Geometry: final body of the model. Coordinates: model frame, mm. A direction names the side the tool comes from. Round coordinates to 2 decimals unless told otherwise and drop trailing zeros. Write each loop counter-clockwise with the first axis right and the second up, starting at its lowest first coordinate (ties: lowest second). Pieces come first, ordered by that corner, then holes. Notation, with made-up numbers: M 6,59.5 L 41,59.5 A33 cw 41,88.5 Z; hole C 79.5,26 d5. An arc over 180 degrees is marked long. Answer as CSV lines item,"result". Start each with the question number.
Q1. Section query D-D on x = 121.5. Output: boundary loops of the cut face in (y, z), and give its area (3 significant figures).
Q2. Section query A-A on z = -21. Output: boundary loops of the cut face in (x, y) (3 decimals), and give its area (3 significant figures).
Q3. Ray query, probe 1 along Z at (x, y) = (28.5, 13); probe 2 along Z at (x, y) = (79, 8.5); probe 3 along Z at (x, y) = (153.5, 21.5). Return the intervals inside material, ascending.
Q4. Reachability of faces 1 (the cylindrical face through (196.46, 3.22, -65.56)), 2 (the flat face through (27, 13, -69.85)) from +Z, -Z, +X, -X, +Y, -Y: full face, straight path, thin tool, end or side. Return the list, or none.
Q5. Mould query, pull axis Z, two halves, no side actions, for faces 3 (the flat face through (92, 13, -76.2)), 4 (the cylindrical face through (-4.404, 18.783, 4.502)), 5 (the flat face through (121, 0, -66)), 6 (the cylindrical face through (183.17, 3.22, -64.18)). Classes: pulls with the +Z half, pulls with the -Z half, needs draft (parallel to the pull), parting line crosses it, or undercut.
Q6. First-contact query: pin 1 (1.5 mm diameter, centred on x = 143.5, z = -72.5, fed in from +Y); pin 2 (1.5 mm diameter, centred on x = 122, z = -76.5, fed in from +Y). Flat tips, straight axial feed; report the tip coordinate or a pass-through.
Q7. Section query C-C on x = 206. Output: boundary loops of the cut face in (y, z), and give its area (3 significant figures).
Autodesk Inventor part; units mm, degrees
ref_plane "YZ Plane" through (0, 0, 0) normal (1, 0, 0) x (0, 1, 0)
ref_plane "XZ Plane" through (0, 0, 0) normal (0, 1, 0) x (-1, 0, 0)
ref_plane "XY Plane" through (0, 0, 0) normal (0, 0, 1) x (1, 0, 0)
sketch "Sketch1" plane through (0, 0, 0) normal (0, 1, 0) x (-1, 0, 0)
  line L0 (0, 0) -> (-238.125, 0)
  line L1 (-238.125, 0) -> (-238.125, -133.35)
  line L2 (-238.125, -133.35) -> (0, -133.35)
  line L3 (0, -133.35) -> (0, 0)
  line L4 (0, 6.35) -> (-237.998, 6.35)
  line L5 (-244.475, -0.127) -> (-244.475, -133.35)
  line L6 (-238.125, -139.7) -> (-0.1245, -139.7)
  line L7 (6.35, -133.35) -> (6.35, 0)
  arc A0 (-0.1245, -139.7) -> (6.35, -133.35) centre (-0.1245, -133.2243) ccw
  arc A1 (6.35, 0) -> (-0.1245, 6.35) centre (-0.1258, -0.127) ccw
  arc A2 (-244.475, -133.2243) -> (-238.125, -139.7) centre (-237.998, -133.2242) ccw
  arc A3 (-237.998, 6.35) -> (-244.475, -0.127) centre (-237.998, -0.127) ccw
  dimension "d0" = 238.125
  dimension "d1" = 133.35
  dimension "d2" = 6.35
  dimension "d9" = 6.477
  dimension "d10" = 6.477
  dimension "d11" = 6.477
extrude "Extrusion1" add sketch "Sketch1" along normal blind 38.1
sketch "Sketch2" plane through (0, 0, 0) normal (0, -1, 0) x (1, 0, 0)
  line L0 (0, 0) -> (238.125, 0)
  line L1 (238.125, 0) -> (238.125, -133.35)
  line L2 (238.125, -133.35) -> (0, -133.35)
  line L3 (0, -133.35) -> (0, 0)
  dimension "d5" = 238.125
  dimension "d6" = 133.35
extrude "Extrusion2" add sketch "Sketch2" against normal blind 6.35
sketch "Sketch7" plane through (0, 6.35, 0) normal (0, 1, 0) x (1, 0, 0)
  line L0 (237.998, 0) -> (155.448, 0)
  line L1 (238.125, 0) -> (0, 0)
  line L2 (155.448, 0) -> (155.448, 57.15)
  line L3 (155.448, 57.15) -> (237.998, 57.15)
  circle A0 centre (218.3382, 65.3946) radius 3.175
  circle A1 centre (199.6313, 65.4249) radius 3.175
  line L4 (218.3382, 65.3946) -> (180.2382, 65.3946)
  circle A2 centre (180.2382, 65.3946) radius 3.175
  dimension "d31" = 82.55
  dimension "d32" = 57.15
  dimension "d33" = 6.35
  dimension "d36" = 6.35
  dimension "d37" = 38.1
  dimension "d38" = 6.35
extrude "Extrusion4" cut sketch "Sketch7" against normal blind 6.35
sketch "Sketch11" plane through (0, 6.35, 0) normal (0, 1, 0) x (1, 0, 0)
  line L0 (57.15, 78.6953) -> (0, 78.6953)
  line L1 (47.625, 76.2) -> (127, 76.2)
  line L2 (47.625, 76.2) -> (127, 76.2)
  line L3 (127, 76.2) -> (127, 63.5)
  line L4 (127, 63.5) -> (47.625, 63.5)
  line L5 (47.625, 63.5) -> (47.625, 76.2)
  line L6 (114.4338, 63.5) -> (127.1338, 63.5)
  line L7 (127.1338, 63.5) -> (127.1338, 0)
  line L8 (127.1338, 0) -> (114.4338, 0)
  line L9 (114.4338, 0) -> (114.4338, 63.5)
  line L10 (238.125, 0) -> (0, 0)
  line L11 (0, 0) -> (0, 82.55)
  line L12 (0, 0) -> (0, 133.35)
  line L13 (0, 82.55) -> (57.15, 82.55)
  line L14 (57.15, 82.55) -> (57.15, 0)
  line L15 (0, 78.6953) -> (47.625, 78.6953)
  line L16 (47.625, 78.6953) -> (47.625, 69.85)
  line L17 (47.625, 69.85) -> (0, 69.85)
  line L18 (0, 69.85) -> (0, 78.6953)
  line L19 (57.15, 78.6953) -> (0, 78.6953)
  line L20 (0, 78.6953) -> (0, 85.0453)
  line L21 (0, 85.0453) -> (57.15, 85.0453)
  line L22 (57.15, 85.0453) -> (57.15, 78.6953)
  point P0 (0, 97.7453)
  point P1 (0, 69.85)
  dimension "d59" = 79.375
  dimension "d60" = 12.7
  dimension "d61" = 12.7
  dimension "d62" = 63.5
  dimension "d70" = 82.55
  dimension "d71" = 6.35
extrude "Extrusion7" add sketch "Sketch11" along normal blind 12.7 contours L0 L11 L13 L14 | L16 L5 L17 L11 L0 | L13 L12 L21 L22 | L14 L4 L5 L1 | L1 L3 L4 L14 | L6 L7 L8 L9 L4
sketch "Sketch12" plane through (0, 6.35, 0) normal (0, 1, 0) x (1, 0, 0)
  line L0 (238.125, 0) -> (0, 0)
  line L1 (238.125, 0) -> (155.575, 0)
  line L2 (151.6176, 0) -> (151.6176, 57.15)
  line L3 (155.575, 57.15) -> (238.125, 57.15)
  line L4 (238.125, 57.15) -> (238.125, 0)
  line L5 (151.6176, 0) -> (138.9176, 0)
  line L6 (138.9176, 0) -> (138.9176, 57.15)
  line L7 (138.9176, 57.15) -> (151.6176, 57.15)
  line L8 (155.575, 57.15) -> (155.575, 0)
  point P0 (151.6176, 57.15)
  point P1 (151.6176, 0)
  dimension "d65" = 82.55
  dimension "d66" = 57.15
  dimension "d67" = 12.7
extrude "Extrusion8" add sketch "Sketch12" along normal blind 12.7 contours L0 L6 L7 L2
sketch "Sketch13" plane through (0, 19.05, 0) normal (0, 1, 0) x (1, 0, 0)
  line L0 (0, 85.0453) -> (57.15, 85.0453)
  line L1 (47.625, 69.85) -> (0, 69.85)
  line L2 (0, 85.0453) -> (6.35, 85.0453)
  line L3 (6.35, 85.0453) -> (6.35, 69.85)
  line L4 (6.35, 69.85) -> (0, 69.85)
  line L5 (0, 69.85) -> (0, 85.0453)
  point P0 (0, 0)
  dimension "d72" = 6.35
extrude "Extrusion9" cut sketch "Sketch13" against normal blind 12.7
sketch "Sketch14" plane through (0, 19.05, 0) normal (0, 1, 0) x (1, 0, 0)
  line L0 (47.625, 78.6953) -> (47.625, 76.2)
  line L1 (47.625, 78.6953) -> (57.15, 78.6953)
  line L2 (57.15, 78.6953) -> (57.15, 76.0675)
  line L3 (57.15, 76.0675) -> (47.625, 76.0675)
  line L4 (47.625, 76.0675) -> (47.625, 78.6953)
  point P0 (0, 0)
extrude "Extrusion10" add sketch "Sketch14" against normal blind 12.7
sketch "Sketch15" plane through (0, 19.05, 0) normal (0, 1, 0) x (1, 0, 0)
  point P0 (0, 0)
equation "\"d34\" = d38"
properties part number "SimpleElectronicBox"
Entries:
1,outline,"M 0,-139.7 L 38.1,-139.7 L 38.1,-133.35 L 6.35,-133.35 L 6.35,-76.2 L 19.05,-76.2 L 19.05,0 L 38.1,0 L 38.1,6.35 L 0,6.35 Z"
1,area,"2,300 mm^2"
2,outline,"M -6.35,0 L 244.475,0 L 244.475,38.1 L 238.125,38.1 L 238.125,6.35 L 151.618,6.35 L 151.618,19.05 L 138.918,19.05 L 138.918,6.35 L 127.134,6.35 L 127.134,19.05 L 114.434,19.05 L 114.434,6.35 L 0,6.35 L 0,38.1 L -6.35,38.1 Z"
2,area,"2,320 mm^2"
3,probe 1,"z = -139.7 to -133.35, -85.05 to -69.85, 0 to 6.35"
3,probe 2,"z = -139.7 to -133.35, -76.2 to -63.5, 0 to 6.35"
3,probe 3,"z = -139.7 to -133.35, 0 to 6.35"
4,face 1,"+Y, -Y"
4,face 2,"+Y"
5,face 3,"undercut"
5,face 4,"pulls with the +Z half"
5,face 5,"needs draft"
5,face 6,"undercut"
6,pin 1,"stops at y = 6.35"
6,pin 2,"stops at y = 19.05"
7,outline,"M 0,-139.7 L 38.1,-139.7 L 38.1,-133.35 L 6.35,-133.35 L 6.35,0 L 38.1,0 L 38.1,6.35 L 0,6.35 Z"
7,area,"1,330 mm^2"
